Geometry: final body of the model. Coordinates: model frame, mm. Face numbers are marked on the shaded views. A direction names the side the tool comes from. Round coordinates to 2 decimals unless told otherwise and drop trailing zeros. Loops run counter-clockwise (first coordinate to the right, second up) from the corner with the lowest first, then second, coordinate; pieces in that order, holes last. Notation, with made-up numbers: (5.25, 1.25) - (10.25, 1.25) arc R7 ccw to (10.25, 9.25) - close; hole circle Ø1 at (32, 63.5). An arc over 180 degrees is marked (long way). Answer as CSV lines item,"result".
from build123d import *

# Parameters (mm, degrees)
SKETCH_1_W      = 88
SKETCH_1_H      = 10
SKETCH_3_W      = 5
SKETCH_3_H      = 60
SKETCH_4_W      = 30
SKETCH_4_H      = 30
EXTRUDE_1_DEPTH = 25


with BuildPart() as part:
    # 草图1 → 旋转1 (revolve)
    with BuildSketch(Plane.XY, mode=Mode.PRIVATE) as revolve_1_sk:
        Rectangle(SKETCH_1_W, SKETCH_1_H)
    revolve(revolve_1_sk.sketch.rotate(Axis((-44, -5, 0), (1, 0, 0)), 90), axis=Axis((-44, -5, 0), (1, 0, 0)))

    # 草图3 → 旋转2 (revolve)
    with BuildSketch(Plane.XY, mode=Mode.PRIVATE) as revolve_2_sk:
        with Locations((2.5, -5)):
            Rectangle(SKETCH_3_W, SKETCH_3_H)
    revolve(revolve_2_sk.sketch.rotate(Axis((0, -35, 0), (0, 1, 0)), 90), axis=Axis((0, -35, 0), (0, 1, 0)))

    # 草图4 → 凸台-拉伸1 (add, symmetric)
    with BuildSketch(Plane(origin=(0, 0, 0), x_dir=(0, 0, -1), z_dir=(1, 0, 0))):
        with Locations((0, -5)):
            Rectangle(SKETCH_4_W, SKETCH_4_H)
    extrude(amount=EXTRUDE_1_DEPTH, both=True)


solid = part.part
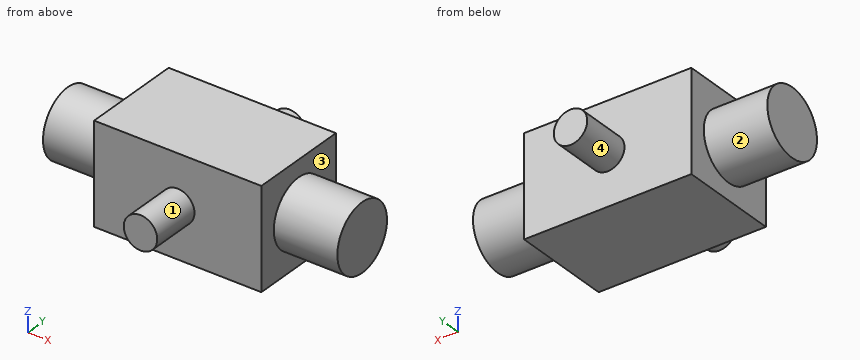
(1) Pin query (flat end, axial travel): P1, Ø6, axis at x = 3.5, y = 15.5, coming from the +Z side; P2, Ø2, axis at x = 5.5, z = -9.5, coming from the +Y side; P3, Ø1.5, axis at x = -17, z = -7.5, coming from the -Y side. Return the tip coordinate at first contact, or that it passes through.
Findings below:
P1,"z = 4.97"
P2,"y = 10"
P3,"y = -20"
(2) Section B-B (x = 0). Output: boundary loops of the cut face in (y, z).
Findings below:
outline,"(-35, -5) - (-20, -5) - (-20, -15) - (10, -15) - (10, -5) - (25, -5) - (25, 5) - (10, 5) - (10, 15) - (-20, 15) - (-20, 5) - (-35, 5) - close"
(3) Material intervals for line 1 along Y through (x, z) = (-8, 4); line 2 along X through (y, z) = (8, 9.5); line 3 along X through (y, z) = (-30, -0.25), sorted ascending.
Findings below:
line 1,"-20 to 10"
line 2,"-25 to 25"
line 3,"-4.99 to 4.99"
(4) Section C-C (z = -2). Output: boundary loops of the cut face in (x, y).
Findings below:
outline,"(-44, -14.8) - (-25, -14.8) - (-25, -20) - (-4.58, -20) - (-4.58, -35) - (4.58, -35) - (4.58, -20) - (25, -20) - (25, -14.8) - (44, -14.8) - (44, 4.8) - (25, 4.8) - (25, 10) - (4.58, 10) - (4.58, 25) - (-4.58, 25) - (-4.58, 10) - (-25, 10) - (-25, 4.8) - (-44, 4.8) - close"
(5) Access query for the marked faces 1, 2, 3 and 4. Directions: +Z, -Z, +X, -X, +Y, -Y. A direction counts if a zero-diameter tool reaches every point of the face in a straight line with its end or side. Return the directions, or none.
Findings below:
face 1,"-Y"
face 2,"-X"
face 3,"+X"
face 4,"+Y"
(6) Section A-A (y = -5). Output: boundary loops of the cut face in (x, z).
Findings below:
outline,"(-44, -10) - (-25, -10) - (-25, -15) - (25, -15) - (25, -10) - (44, -10) - (44, 10) - (25, 10) - (25, 15) - (-25, 15) - (-25, 10) - (-44, 10) - close"
(7) Section D-D (y = -19). Output: boundary loops of the cut face in (x, z).
Findings below:
outline,"(-25, -15) - (25, -15) - (25, 15) - (-25, 15) - close"
